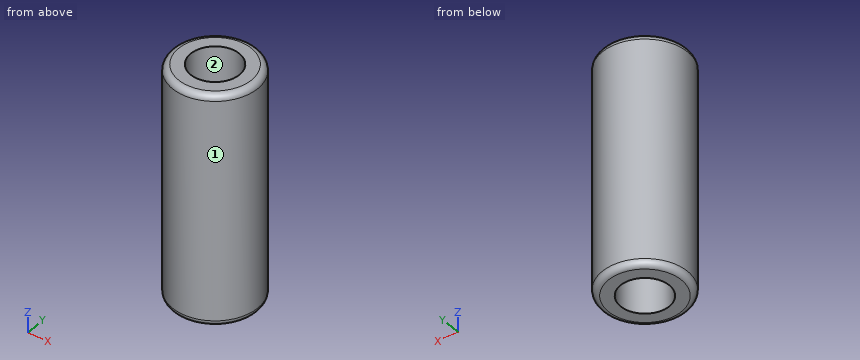
```python
from build123d import *

# Parameters (mm, degrees)
F0_R     = 10.5
F1_DEPTH = 57
F2_R     = 6.01
F3_DEPTH = 57.001
F4_R     = 1.5


with BuildPart() as f1:
    # F0 (on Top) → F1 (new body)
    with BuildSketch(Plane.XY):
        Circle(F0_R)
    extrude(amount=F1_DEPTH)

    # F2 (on face) → F3 (cut, through all)
    with BuildSketch(Plane.XY.offset(57)):
        Circle(F2_R)
    extrude(amount=-F3_DEPTH, mode=Mode.SUBTRACT)

    # F4
    f4_edges = [f1.edges().sort_by_distance(p)[0] for p in [
        (-10.5, 0, 57),
        (-10.5, 0, 0),
    ]]
    fillet(f4_edges, radius=F4_R)


solid = f1.part
```
Input: part model. Units: mm. Frame: model coordinates. Face numbers are marked on the shaded views. Give positions to 0.01 mm unless a question says otherwise; leave off trailing zeros. Order: outer loops, then holes, each group sorted by start corner. A loop starts at its lowest first (then second) coordinate and runs counter-clockwise, first axis right, second up. Notation, with made-up numbers: (-9.5, 50) -> (-3.5, 50) arc R16 cw to (-3.5, 80) -> close; hole circle Ø7 at (16, -22). An arc over 180 degrees is marked (long way). Write each question's results on one line, items separated by ' | '. Start each with the question number.
Item 1: Line query: line 1 (Y direction, x = 0, z = 39.5); line 2 (Y direction, x = 3, z = 27.5); line 3 (X direction, y = -5.5, z = 52). Output: solid intervals per line, ascending.
Item 2: Mould query, pull axis Y, two halves, no side actions, for the marked faces 1 and 2. Classes: pulls with the +Y half, pulls with the -Y half, needs draft (parallel to the pull), parting line crosses it, or undercut.
Item 3: Cut plane C-C on z = 49.5. Return the cut outline in (x, y), then the cut area to 3 significant figures.
Item 4: Contact query for flat-ended pins moving along their axis: P1, Ø4, axis at x = -1.5, y = -1.5, coming from the -Z side; P2, Ø6, axis at y = 6.5, z = 23, coming from the -X side; P3, Ø4, axis at y = 3.5, z = 28, coming from the -X side. Output: stop coordinate, or through.
Item 5: Cut plane A-A on y = 0. Return the cut outline in (x, z), then the cut area to 3 significant figures.
Established:
1) line 1: -10.5 to -6.01, 6.01 to 10.5 | line 2: -10.06 to -5.21, 5.21 to 10.06 | line 3: -8.94 to -2.42, 2.42 to 8.94
2) face 1: parting line crosses it | face 2: undercut
3) outline: circle Ø21 at (0, 0); hole circle Ø12.02 at (0, 0) | area: 233 mm^2
4) P1: through | P2: x = -9.9 | P3: x = -10.39
5) outline: (-10.5, 1.5) arc R1.5 ccw to (-9, 0) -> (-6.01, 0) -> (-6.01, 57) -> (-9, 57) arc R1.5 ccw to (-10.5, 55.5) -> close; (6.01, 0) -> (9, 0) arc R1.5 ccw to (10.5, 1.5) -> (10.5, 55.5) arc R1.5 ccw to (9, 57) -> (6.01, 57) -> close | area: 510 mm^2
